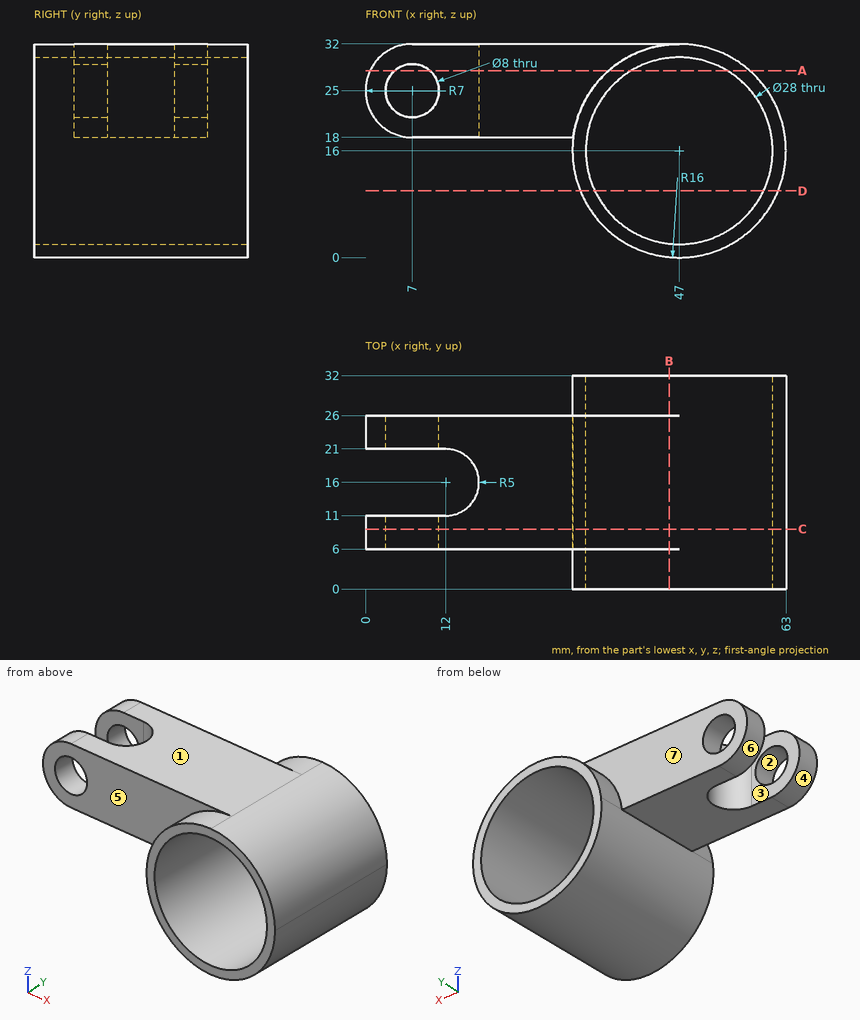
Study the drawing (mm; zero at the part's minimum x, y, z) and answer. A direction names the side the tool comes from. Coordinates: 2 decimals unless noted, no trailing zeros. Write each loop counter-clockwise with the first axis right and the second up, starting at its lowest first coordinate (ties: lowest second). Pieces come first, ordered by that corner, then holes. Notation, with made-up numbers: (-23, 81.5) - (24, 81.5) arc R17 ccw to (24, 106.5) - close; hole circle Ø5 at (12, 15). An arc over 180 degrees is marked (long way). Return JSON: item names as keys, results as strings. Group by question number.
1. A cutting plane is placed at C-C, the plane y = 9. Determine the outline of the cut face in (x, z), plus the area to 3 significant figures.
2. A cutting plane is placed at D-D, the plane z = 10. Determine the outline of the cut face in (x, y).
3. Given pin 1 (6 mm diameter, centred on x = 6.5, z = 23, fed in from -Y); pin 2 (13 mm diameter, centred on x = 7, z = 21.5, fed in from +Y); pin 3 (12 mm diameter, centred on x = 29.5, y = 28.5, fed in from -Z), each flat-ended and moving along its own axis, determine where each tip first touches the part or whether it passes through.
4. A cutting plane is placed at A-A, the plane z = 28. Determine the outline of the cut face in (x, y), plus the area to 3 significant figures.
5. A cutting plane is placed at B-B, the plane x = 45.5. Determine the outline of the cut face in (y, z), plus the area to 3 significant figures.
6. Determine the mould class of the marked faces 1, 2, 3 and 4 for opening direction Z: released by +Z, released by -Z, zero draft, split by the parting line, or undercut.
7. Straight lines are drawn through the part: L1, parallel to X at y = 14, z = 16; L2, parallel to Z at x = 7, y = 23.2; L3, parallel to X at y = 9, z = 25. For each, find the intervals that lie inside material, in ascending order.
8. Which of the six approach directions +Z, -Z, +X, -X, +Y, -Y give full straight-line access (tool end or side, diameter ignored) to the marked faces 5, 6 and 7?
Ans:
{
 "1": {"outline": "(7, 18) - (31.13, 18) arc R16 ccw (long way) to (63, 16) arc R16 ccw to (47, 32) - (7, 32) arc R7 ccw to start; hole circle Ø8 at (7, 25); hole circle Ø28 at (47, 16)", "area": "606 mm²"},
 "2": {"outline": "(32.17, 0) - (34.35, 0) - (34.35, 32) - (32.17, 32) - close; (59.65, 0) - (61.83, 0) - (61.83, 32) - (59.65, 32) - close"},
 "3": {"pin 1": "y = 6", "pin 2": "y = 26", "pin 3": "z = 4.88"},
 "4": {"outline": "(0.68, 6) - (4.35, 6) - (4.35, 11) - (0.68, 11) - close; (0.68, 21) - (4.35, 21) - (4.35, 26) - (0.68, 26) - close; (9.65, 6) - (36.42, 6) - (36.42, 0) - (39.79, 0) - (39.79, 32) - (36.42, 32) - (36.42, 26) - (9.65, 26) - (9.65, 21) - (12, 21) arc R5 cw to (12, 11) - (9.65, 11) - close; (54.21, 0) - (57.58, 0) - (57.58, 32) - (54.21, 32) - close", "area": "725 mm²"},
 "5": {"outline": "(0, 0.07) - (32, 0.07) - (32, 2.08) - (0, 2.08) - close; (0, 29.92) - (32, 29.92) - (32, 31.93) - (26, 31.93) - (26, 32) - (6, 32) - (6, 31.93) - (0, 31.93) - close", "area": "130 mm²"},
 "6": {"face 1": "released by +Z", "face 2": "undercut", "face 3": "zero draft", "face 4": "split by the parting line"},
 "7": {"L1": "31 to 33, 61 to 63", "L2": "18 to 21, 29 to 32", "L3": "0 to 3, 11 to 36.28, 57.72 to 60.23"},
 "8": {"face 5": "+Z, -X, -Y", "face 6": "-X, +Y, -Y", "face 7": "+Z, -X, +Y"}
}
